Read the model definition and answer for the solid it produces. Units are mm, in the model's axes. A direction names the side the tool comes from. Coordinates: 2 decimals unless noted, no trailing zeros. Order: outer loops, then holes, each group sorted by start corner. A loop starts at its lowest first (then second) coordinate and runs counter-clockwise, first axis right, second up. Notation, with made-up numbers: M -28.75,54.5 L 21.25,54.5 A21 ccw 21.25,70.5 Z; hole C 85,7.5 d6. An arc over 180 degrees is marked long. Use a Markdown table: item, result. Add a question column.
1) Each of these flat-tipped pins is pushed along its axis until it touches: pin 1 Ø1 at (y, z) = (-51, -0.5) entering from +X; pin 2 Ø2 at (x, y) = (8, 0) entering from -Z (3 decimals); pin 3 Ø4 at (x, y) = (2, -24) entering from +Z; pin 4 Ø1.3 at (x, y) = (6.5, -66) entering from -Z. Where does it stop, or does it pass through?
2) Find section A-A on x = 0. Write down the section's boundary in (y, z).
3) Find section B-B on y = -21. Write down the section's boundary in (x, z), plus the area to 3 significant figures.
4) The mould has two halves that part along X. Classify faces 4 (the face through (11, -30, -2)), 5 (the face through (-9.2, 0.05, -0.37)), 6 (the face through (0.2, -11, -0.4)): released by +X, released by -X, zero draft, split by the parting line, or undercut.
5) For faces 1 (the face through (-2.38, -70.74, -1.43)), 2 (the face through (-7, -53, -2.35)), 3 (the face through (-5.8, -64.5, -1.2)), determine the directions among +Z, -Z, +X, -X, +Y, -Y from which every point of the face is accessible in a straight line to the end or side of a thin tool.
6) Find the intervals of material crossed by probe 1 along Y at (x, z) = (-1, -3.3); probe 2 along X at (y, z) = (-53, -2.55); probe 3 along Y at (x, z) = (5, -2.4), in increasing order. Write a range as [from, to].
from build123d import *

# Parameters (mm, degrees)
RESSALTO_EXTRUS_O1_DEPTH                             = 0.75
RESSALTO_EXTRUS_O2_DEPTH                             = 3
REBAIXO_PARA_SHCS_M21_D                              = 2.4
REBAIXO_PARA_SHCS_M21_CBORE_D                        = 4.4
REBAIXO_PARA_SHCS_M21_CBORE_DEPTH                    = 3
RESSALTO_EXTRUS_O3_START                             = 0.75
ESBO_O4_R                                            = 11
RESSALTO_EXTRUS_O3_DEPTH                             = 0.75
ESBO_O5_R                                            = 3.05
CORTE_EXTRUS_O1_DEPTH                                = 72.944857356
REBAIXO_PARA_PARAFUSO_COM_CABE_A_REDONDA_D           = 2.4
REBAIXO_PARA_PARAFUSO_COM_CABE_A_REDONDA_CBORE_D     = 4.4
REBAIXO_PARA_PARAFUSO_COM_CABE_A_REDONDA_CBORE_DEPTH = 1.4
PADR_OCIRCULAR1_COUNT                                = 4


with BuildPart() as part:
    # Esboço1 → Ressalto-extrusão1 (new body)
    with BuildSketch(Plane.XY):
        with BuildLine():
            ThreePointArc((-4.5, 0), (0, -4.5), (4.5, 0))
            ThreePointArc((4.5, 0), (7.75, 3.25), (11, 0))
            ThreePointArc((11, 0), (0, -11), (-11, 0))
            ThreePointArc((-11, 0), (-7.75, 3.25), (-4.5, 0))
        make_face()
    extrude(amount=-RESSALTO_EXTRUS_O1_DEPTH)

    # Esboço3 → Ressalto-extrusão2 (add)
    with BuildSketch(Plane(origin=(0, 0, -0.75), x_dir=(-1, 0, 0), z_dir=(0, 0, -1))):
        with BuildLine():
            Line((-11, 0), (-11, -60))
            ThreePointArc((-11, -60), (0, -71), (11, -60))
            Line((11, -60), (11, 0))
            ThreePointArc((11, 0), (7.75, 3.25), (4.5, 0))
            ThreePointArc((4.5, 0), (0, -4.5), (-4.5, 0))
            ThreePointArc((-4.5, 0), (-7.75, 3.25), (-11, 0))
        make_face()
    extrude(amount=RESSALTO_EXTRUS_O2_DEPTH)

    # Rebaixo para SHCS M21 (through all)
    with Locations(Plane(origin=(0, 0, -3.75), x_dir=(-1, 0, 0), z_dir=(0, 0, -1))):
        with Locations((-8, 0), (-5.656854249, -5.656854249), (0, -8), (5.656854249, -5.656854249), (8, 0)):
            CounterBoreHole(REBAIXO_PARA_SHCS_M21_D / 2, REBAIXO_PARA_SHCS_M21_CBORE_D / 2, REBAIXO_PARA_SHCS_M21_CBORE_DEPTH)

    # Esboço4 → Ressalto-extrusão3 (add)
    with BuildSketch(Plane.XY.offset(-0.75).offset(RESSALTO_EXTRUS_O3_START)):
        with Locations((0, -60)):
            Circle(ESBO_O4_R)
    extrude(amount=-RESSALTO_EXTRUS_O3_DEPTH)

    # Esboço5 → Corte-extrusão1 (cut, through all)
    with BuildSketch(Plane(origin=(0, 0, -3.75), x_dir=(-1, 0, 0), z_dir=(0, 0, -1))):
        with Locations((0, -60)):
            Circle(ESBO_O5_R)
    extrude(amount=-CORTE_EXTRUS_O1_DEPTH, mode=Mode.SUBTRACT)

    # Rebaixo para parafuso com cabeça redonda de M21 (through all)
    with Locations(Plane(origin=(0, 0, -3.75), x_dir=(-1, 0, 0), z_dir=(0, 0, -1))):
        with Locations((5.624741587, -65.688785642)):
            rebaixo_para_parafuso_com_cabe_a_redonda = CounterBoreHole(REBAIXO_PARA_PARAFUSO_COM_CABE_A_REDONDA_D / 2, REBAIXO_PARA_PARAFUSO_COM_CABE_A_REDONDA_CBORE_D / 2, REBAIXO_PARA_PARAFUSO_COM_CABE_A_REDONDA_CBORE_DEPTH)

    # PadrãoCircular1: Rebaixo para parafuso com cabeça redonda de M21 ×4 about axis
    padr_ocircular1_axis = Axis((0, -60, 0), (0, 0, 1))
    for i in range(1, PADR_OCIRCULAR1_COUNT):
        add(rebaixo_para_parafuso_com_cabe_a_redonda.rotate(padr_ocircular1_axis, i * 360 / PADR_OCIRCULAR1_COUNT), mode=Mode.SUBTRACT)


solid = part.part
Check result:
| question | item | result |
|---|---|---|
| 1 | pin 1 | stops at x = 11 |
| 1 | pin 2 | passes through |
| 1 | pin 3 | stops at z = -0.75 |
| 1 | pin 4 | stops at z = -2.35 |
| 2 | outline | M -71,-3.75 L -63.05,-3.75 L -63.05,0 L -71,0 Z; M -56.95,-3.75 L -10.2,-3.75 L -10.2,-0.75 L -9.2,-0.75 L -9.2,0 L -11,0 L -11,-0.75 L -49,-0.75 L -49,0 L -56.95,0 Z; M -6.8,-0.75 L -5.8,-0.75 L -5.8,-3.75 L -4.5,-3.75 L -4.5,0 L -6.8,0 Z |
| 3 | outline | M -11,-3.75 L 11,-3.75 L 11,-0.75 L -11,-0.75 Z |
| 3 | area | 66.0 mm2 |
| 4 | face 4 | released by +X |
| 4 | face 5 | undercut |
| 4 | face 6 | split by the parting line |
| 5 | face 1 | +Z |
| 5 | face 2 | -Z |
| 5 | face 3 | +Z, -Z |
| 6 | probe 1 | y = [-70.95, -62.88], [-57.12, -9.96], [-6.04, -4.39] |
| 6 | probe 2 | x = [-11, -7.41], [-3.97, 3.86], [7.39, 11] |
| 6 | probe 3 | y = [-69.8, -67.71], [-63.54, -56.42], [-52.2, -7.76], [-3.56, 1.73] |
